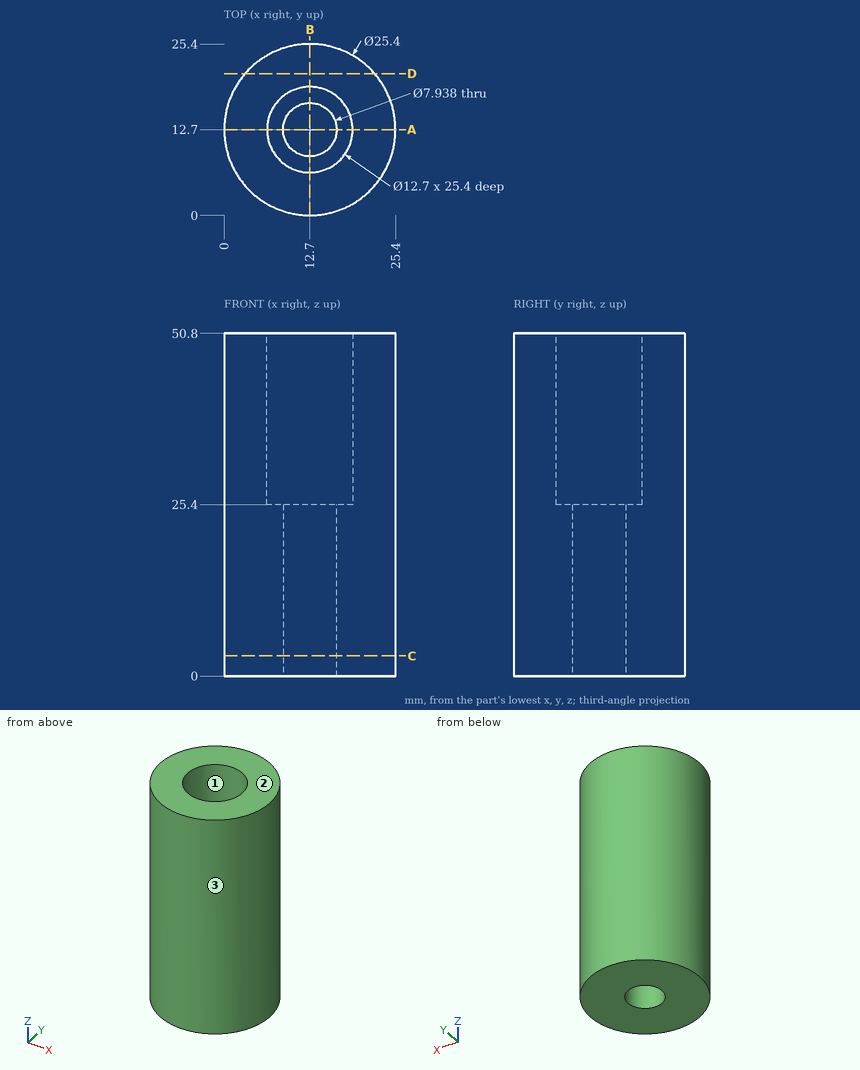
Verification items for this drawing (mm, ordinates from the low corner). Coordinates: 2 decimals unless noted, no trailing zeros. Loops run counter-clockwise (first coordinate to the right, second up) from the corner with the lowest first, then second, coordinate; pieces in that order, holes last. Notation, with made-up numbers: (-13, 66) - (19, 66) arc R6 ccw to (19, 75) - close; hole circle Ø7 at (-31.75, 66.25). An arc over 180 degrees is marked (long way). One line per item, written item: value. Start each with the question number.
(1) Material ranges on line 1 (Y direction, x = 12.7, z = 5.5); line 2 (Y direction, x = 12.7, z = 45.5); line 3 (X direction, y = 11.25, z = 11.5) (1 decimal), recorded low to high. Write a range as [from, to].
(2) Depth check by flat-ended pin: P1, Ø10, axis at y = 21, z = 16, coming from the +X side; P2, Ø4, axis at y = 5.5, z = 35, coming from the +X side; P3, Ø3, axis at x = 19, z = 22.5, coming from the +Y side; P4, Ø7, axis at x = 12.7, y = 12.7, coming from the +Z side. Enter the tip coordinate at first touch or a pass-through.
(3) Cross-section at D-D on y = 21. Enter the section's corners in (x, z).
(4) Cross-section at C-C on z = 3. Enter the section's corners in (x, y).
(5) Mould release check, pull along X, two halves, no side actions. Record for the marked faces 1, 2 and 3: released by +X, released by -X, zero draft, split by the parting line, or undercut.
(6) Cross-section at A-A on y = 12.7. Enter the section's corners in (x, z).
Results below:
1. line 1: y = [0, 8.73], [16.67, 25.4]
1. line 2: y = [0, 6.35], [19.05, 25.4]
1. line 3: x = [0.1, 9], [16.4, 25.3]
2. P1: stops at x = 24.96
2. P2: stops at x = 24.29
2. P3: stops at y = 24.46
2. P4: passes through
3. outline: (3.09, 0) - (22.31, 0) - (22.31, 50.8) - (3.09, 50.8) - close
4. outline: circle Ø25.4 at (12.7, 12.7); hole circle Ø7.94 at (12.7, 12.7)
5. face 1: undercut
5. face 2: zero draft
5. face 3: split by the parting line
6. outline: (0, 0) - (8.73, 0) - (8.73, 25.4) - (6.35, 25.4) - (6.35, 50.8) - (0, 50.8) - close; (16.67, 0) - (25.4, 0) - (25.4, 50.8) - (19.05, 50.8) - (19.05, 25.4) - (16.67, 25.4) - close
